The model under review builds one solid part; all positions refer to its coordinate system, in mm. A direction names the side the tool comes from. Coordinates: 2 decimals unless noted, no trailing zeros. Loops run counter-clockwise (first coordinate to the right, second up) from the corner with the lowest first, then second, coordinate; pieces in that order, holes last. Notation, with made-up numbers: (60.25, 63) - (80.25, 63) arc R7 ccw to (80.25, 73) - close; hole circle Ø6 at (53, 76). An arc over 180 degrees is marked (long way). One line per item, written item: value. Start each with the question number.
1. We need section D-D, the plane x = -12.5. Count the separate pieces of the cut face and the enclosed holes in it, then the cut area to 3 significant figures.
2. Insertion check: P1, Ø20, axis at x = -7.5, y = 3.5, coming from the -Z side; P2, Ø5, axis at y = -11, z = 6, coming from the -X side; P3, Ø1.9, axis at x = -11.69, y = -6.75, coming from the -Z side. Each pin has a flat end and moves straight along its axis. Give the tip position at first contact, or say it passes through.
3. We need section B-B, the plane x = 0. Give the boundary of the cut face in (y, z), then the cut area to 3 significant figures.
4. Mouldability with a two-part tool opening along Y and no side actions: class faces 1 (the face through (2.17, -9.76, 4.68)), 2 (the face through (7.5, -7.5, 0)), 3 (the face through (-13.887, -10.648, 3.758)) as +Y half, -Y half, draft (parallel to the pull), parting line (faces both ways), or undercut.
5. We need section A-A, the plane y = 0. Give the boundary of the cut face in (x, z), then the cut area to 3 significant figures.
6. To check wall thickness, follow line 1 (Y direction, x = 0, z = 5.75); line 2 (Y direction, x = -11, z = 6); line 3 (X direction, y = -8, z = 2.25). State the ranges of each line that lie inside material, in increasing order.
7. We need section C-C, the plane z = 7. Give the boundary of the cut face in (x, y).
8. For faces 4 (the face through (-4.336, -19.524, 8.546)), 5 (the face through (0, -18, 7.5)), list the 3-axis set-ups (+Z, -Z, +X, -X, +Y, -Y) from which the entire face can be reached by the end or side of a thin tool; tool diameter is ignored.
from build123d import *
from OCP.BRepFilletAPI import BRepFilletAPI_MakeChamfer

# Parameters (mm, degrees)
SKETCH_1_R          = 17.5
SKETCH_1_R_2        = 1.55
EXTRUDE_1_DEPTH     = 7.5
SKETCH_2_R          = 20
SKETCH_2_R_2        = 1.55
EXTRUDE_2_DEPTH     = 2
CHAMFER_1_SIZE      = 0.1
CHAMFER_1_SIZE2     = 0.119175359
SKETCH_4_R          = 10
CUT_EXTRUDE_1_DEPTH = 25


with BuildPart() as part:
    # 草图1 → 凸台-拉伸1 (new body)
    with BuildSketch(Plane.XY):
        Circle(SKETCH_1_R)
        with Locations((0, 13.5)):
            Circle(SKETCH_1_R_2, mode=Mode.SUBTRACT)
        with Locations((11.691342951, 6.75)):
            Circle(SKETCH_1_R_2, mode=Mode.SUBTRACT)
        with Locations((11.691342951, -6.75)):
            Circle(SKETCH_1_R_2, mode=Mode.SUBTRACT)
        with Locations((0, -13.5)):
            Circle(SKETCH_1_R_2, mode=Mode.SUBTRACT)
        with Locations((-11.691342951, -6.75)):
            Circle(SKETCH_1_R_2, mode=Mode.SUBTRACT)
        with Locations((-11.691342951, 6.75)):
            Circle(SKETCH_1_R_2, mode=Mode.SUBTRACT)
    extrude(amount=EXTRUDE_1_DEPTH)

    # 草图2 → 凸台-拉伸2 (add)
    with BuildSketch(Plane.XY.offset(7.5)):
        Circle(SKETCH_2_R)
        with Locations((11.691342951, 6.75)):
            Circle(SKETCH_2_R_2, mode=Mode.SUBTRACT)
        with Locations((11.691342951, -6.75)):
            Circle(SKETCH_2_R_2, mode=Mode.SUBTRACT)
        with Locations((0, -13.5)):
            Circle(SKETCH_2_R_2, mode=Mode.SUBTRACT)
        with Locations((-11.691342951, -6.75)):
            Circle(SKETCH_2_R_2, mode=Mode.SUBTRACT)
        with Locations((-11.691342951, 6.75)):
            Circle(SKETCH_2_R_2, mode=Mode.SUBTRACT)
        with Locations((0, 13.5)):
            Circle(SKETCH_2_R_2, mode=Mode.SUBTRACT)
    extrude(amount=EXTRUDE_2_DEPTH)

    # 倒角1: one chamfer whose edges measure the first distance from different faces: ONE call of the kernel's chamfer builder (chamfer() names one face for all edges)
    chamfer_1_edges_1 = [part.edges().sort_by_distance(p)[0] for p in [
        (-17.5, 0, 0),
    ]]
    chamfer_1_side_1 = [part.faces().sort_by_distance(p)[0] for p in [
        (0, 0, 0),
    ]]
    chamfer_1_edges_2 = [part.edges().sort_by_distance(p)[0] for p in [
        (-20, 0, 7.5),
    ]]
    chamfer_1_side_2 = [part.faces().sort_by_distance(p)[0] for p in [
        (-19.434314575, 0, 7.5),
    ]]
    chamfer_1 = BRepFilletAPI_MakeChamfer(part.part.solid().wrapped)
    for e in chamfer_1_edges_1:
        chamfer_1.Add(CHAMFER_1_SIZE, CHAMFER_1_SIZE2, e.wrapped, chamfer_1_side_1[0].wrapped)  # the first distance lies on this face
    for e in chamfer_1_edges_2:
        chamfer_1.Add(CHAMFER_1_SIZE, CHAMFER_1_SIZE2, e.wrapped, chamfer_1_side_2[0].wrapped)  # the first distance lies on this face
    add(Compound.cast(chamfer_1.Shape()), mode=Mode.REPLACE)

    # 草图4 → 切除-拉伸1 (cut)
    with BuildSketch(Plane(origin=(0, 0, 0), x_dir=(-1, 0, 0), z_dir=(0, 0, -1))):
        Circle(SKETCH_4_R)
    extrude(amount=-CUT_EXTRUDE_1_DEPTH, mode=Mode.SUBTRACT)


solid = part.part
Findings below:
1. separate pieces: 3
1. enclosed holes: 0
1. area: 196 mm2
2. P1: z = 0
2. P2: x = -17.81
2. P3: through
3. outline: (-20, 7.62) - (-19.9, 7.5) - (-17.5, 7.5) - (-17.5, 0.12) - (-17.4, 0) - (-15.05, 0) - (-15.05, 9.5) - (-20, 9.5) - close; (-11.95, 0) - (-10, 0) - (-10, 9.5) - (-11.95, 9.5) - close; (10, 0) - (11.95, 0) - (11.95, 9.5) - (10, 9.5) - close; (15.05, 0) - (17.4, 0) - (17.5, 0.12) - (17.5, 7.5) - (19.9, 7.5) - (20, 7.62) - (20, 9.5) - (15.05, 9.5) - close
3. area: 93.6 mm2
4. face 1: undercut
4. face 2: draft
4. face 3: parting line
5. outline: (-20, 7.62) - (-19.9, 7.5) - (-17.5, 7.5) - (-17.5, 0.12) - (-17.4, 0) - (-10, 0) - (-10, 9.5) - (-20, 9.5) - close; (10, 0) - (17.4, 0) - (17.5, 0.12) - (17.5, 7.5) - (19.9, 7.5) - (20, 7.62) - (20, 9.5) - (10, 9.5) - close
5. area: 152 mm2
6. line 1: -17.5 to -15.05, -11.95 to -10, 10 to 11.95, 15.05 to 17.5
6. line 2: -13.61 to -8.14, -5.36 to 5.36, 8.14 to 13.61
6. line 3: -15.56 to -12.61, -10.77 to -6, 6 to 10.77, 12.61 to 15.56
7. outline: circle Ø35 at (0, 0); hole circle Ø3.1 at (-11.69, -6.75); hole circle Ø3.1 at (-11.69, 6.75); hole circle Ø20 at (0, 0); hole circle Ø3.1 at (0, -13.5); hole circle Ø3.1 at (0, 13.5); hole circle Ø3.1 at (11.69, -6.75); hole circle Ø3.1 at (11.69, 6.75)
8. face 4: +Z, -Z
8. face 5: -Z
